The listing builds one solid part. Answer for the finished solid, in the listing's coordinates (mm). Face numbers are marked on the shaded views. A direction names the side the tool comes from. Coordinates: 2 decimals unless noted, no trailing zeros. Write each loop counter-clockwise with the first axis right and the second up, starting at its lowest first coordinate (ties: lowest second). Pieces come first, ordered by that corner, then holes. Notation, with made-up numbers: M 65,49.5 L 72,49.5 A6 ccw 72,58.5 Z; hole C 63.5,-7.5 d8. An arc over 180 degrees is marked long. Put each result on its own line as item: value. Start each with the question number.
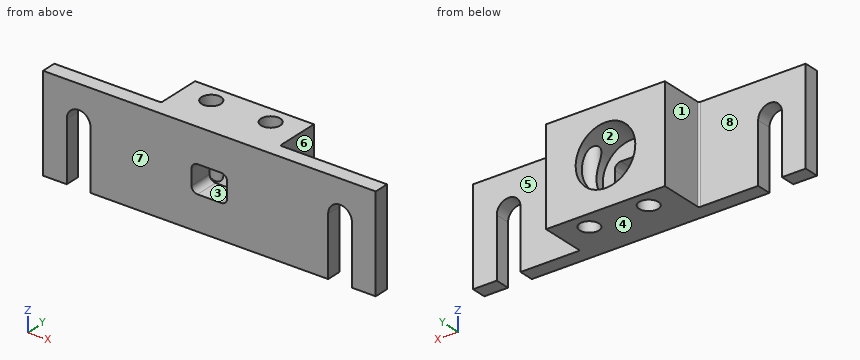
```python
from build123d import *

# Parameters (mm, degrees)
SKETCH1_W           = 28
SKETCH1_H           = 8
BOSS_EXTRUDE1_DEPTH = 1.25
SKETCH2_W           = 10
SKETCH2_H           = 8
BOSS_EXTRUDE2_DEPTH = 3.75
SKETCH3_R           = 2.51
CUT_EXTRUDE1_DEPTH  = 3
SKETCH4_W           = 3
SKETCH4_H           = 2.3
CUT_EXTRUDE2_DEPTH  = 15.866068747
CUT_EXTRUDE4_DEPTH  = 16.035374954
SKETCH7_R           = 0.81
CUT_EXTRUDE5_DEPTH  = 17.881943016
FILLET1_R           = 0.5
FILLET2_R           = 0.127


with BuildPart() as part:
    # Sketch1 → Boss-Extrude1 (new body)
    with BuildSketch(Plane(origin=(0, 0, 0), x_dir=(1, 0, 0), z_dir=(0, 1, 0))):
        Rectangle(SKETCH1_W, SKETCH1_H)
    extrude(amount=BOSS_EXTRUDE1_DEPTH)

    # Sketch2 → Boss-Extrude2 (add)
    with BuildSketch(Plane(origin=(0, 1.25, 0), x_dir=(1, 0, 0), z_dir=(0, 1, 0))):
        Rectangle(SKETCH2_W, SKETCH2_H)
    extrude(amount=BOSS_EXTRUDE2_DEPTH)

    # Sketch3 → Cut-Extrude1 (cut)
    with BuildSketch(Plane(origin=(0, 5, 0), x_dir=(1, 0, 0), z_dir=(0, 1, 0))):
        with Locations(Location((0, 0, 0), (0, 0, 270))):
            Circle(SKETCH3_R)
    extrude(amount=-CUT_EXTRUDE1_DEPTH, mode=Mode.SUBTRACT)

    # Sketch4 → Cut-Extrude2 (cut, through all)
    with BuildSketch(Plane(origin=(0, 2, 0), x_dir=(1, 0, 0), z_dir=(0, 1, 0))):
        Rectangle(SKETCH4_W, SKETCH4_H)
    extrude(amount=-CUT_EXTRUDE2_DEPTH, mode=Mode.SUBTRACT)

    # Sketch6 → Cut-Extrude4 (cut, through all)
    with BuildSketch(Plane(origin=(0, 1.25, 0), x_dir=(1, 0, 0), z_dir=(0, 1, 0))):
        with BuildLine():
            Line((12, 4), (12, -1))
            ThreePointArc((12, -1), (11, -2), (10, -1))
            Line((10, -1), (10, 4))
            Line((10, 4), (12, 4))
        make_face()
        with BuildLine():
            Line((-12, 4), (-12, -1))
            ThreePointArc((-12, -1), (-11, -2), (-10, -1))
            Line((-10, -1), (-10, 4))
            Line((-10, 4), (-12, 4))
        make_face()
    extrude(amount=-CUT_EXTRUDE4_DEPTH, mode=Mode.SUBTRACT)

    # Sketch7 → Cut-Extrude5 (cut, through all)
    with BuildSketch(Plane(origin=(0, 0, -4), x_dir=(-1, 0, 0), z_dir=(0, 0, -1))):
        with Locations((2.5, 3.5)):
            Circle(SKETCH7_R)
    cut_extrude5 = extrude(amount=-CUT_EXTRUDE5_DEPTH, mode=Mode.SUBTRACT)

    # Mirror1: Cut-Extrude5 across plane
    add(cut_extrude5.mirror(Plane.ZY), mode=Mode.SUBTRACT)

    # Fillet1
    fillet1_edges = [part.edges().sort_by_distance(p)[0] for p in [
        (-1.5, 1, -1.15),
        (1.5, 1, -1.15),
        (1.5, 1, 1.15),
        (-1.5, 1, 1.15),
    ]]
    fillet(fillet1_edges, radius=FILLET1_R)

    # Fillet2
    fillet2_edges = [part.edges().sort_by_distance(p)[0] for p in [
        (5, 1.25, 0),
        (-5, 1.25, 0),
    ]]
    fillet(fillet2_edges, radius=FILLET2_R)


solid = part.part
```
1) Determine the mould class of the marked faces 6, 7 and 8 for opening direction Y: +Y half, -Y half, draft (parallel to the pull), parting line (faces both ways), or undercut.
2) A cutting plane is placed at D-D on y = 3.5. Write down the section's boundary in (x, z).
3) Straight lines are drawn through the part: probe 1 along X at (y, z) = (0.35, -1.5); probe 2 along Y at (x, z) = (2.5, 0.5); probe 3 along X at (y, z) = (2.6, 0). For each, find the intervals that lie inside material, in ascending order.
4) For the marked faces 1, 2, 3, 4 and 5, determine the directions among +Z, -Z, +X, -X, +Y, -Y from which every point of the face is accessible in a straight line to the end or side of a thin tool.
5) Given pin 1 Ø3 at (y, z) = (3.5, -1) entering from +X; pin 2 Ø1.3 at (x, y) = (2.5, 3.5) entering from +Z; pin 3 Ø2.5 at (x, z) = (-9.5, 1.5) entering from +Y; pin 4 Ø1.5 at (x, z) = (-1, 0) entering from +Y, each flat-ended and moving along its own axis, determine where each tip first touches the part or whether it passes through.
6) A cutting plane is placed at A-A on z = -2.75. Write down the section's boundary in (x, y), then the cut area to 3 significant figures.
7) A cutting plane is placed at B-B on z = -1.5. Write down the section's boundary in (x, y).
8) A cutting plane is placed at C-C on x = 1.25. Write down the section's boundary in (y, z), then the cut area to 3 significant figures.
Answers follow:
1. face 6: draft
1. face 7: -Y half
1. face 8: +Y half
2. outline: M -5,-4 L -3.31,-4 L -3.31,4 L -5,4 Z; M -1.69,-4 L 1.69,-4 L 1.69,-1.86 A2.51 cw -1.69,-1.86 Z; M -1.69,1.86 A2.51 cw 1.69,1.86 L 1.69,4 L -1.69,4 Z; M 3.31,-4 L 5,-4 L 5,4 L 3.31,4 Z
3. probe 1: x = -14 to -12, -10 to 10, 12 to 14
3. probe 2: y = 0 to 2.69, 4.31 to 5
3. probe 3: x = -5 to -2.51, 2.51 to 5
4. face 1: +Z, -Z, -X, +Y
4. face 2: +Y
4. face 3: +Y, -Y
4. face 4: -Z, +X, -X, +Y, -Y
4. face 5: +Z, -Z, +X, +Y
5. pin 1: stops at x = 5
5. pin 2: passes through
5. pin 3: stops at y = 1.25
5. pin 4: stops at y = 2
6. outline: M -14,0 L -12,0 L -12,1.25 L -14,1.25 Z; M -10,0 L 10,0 L 10,1.25 L 5.13,1.25 A0.13 cw 5,1.38 L 5,5 L -5,5 L -5,1.38 A0.13 cw -5.13,1.25 L -10,1.25 Z; M 12,0 L 14,0 L 14,1.25 L 12,1.25 Z; hole C -2.5,3.5 d1.62; hole C 2.5,3.5 d1.62
6. area: 63.4 mm²
7. outline: M -14,0 L -12,0 L -12,1.25 L -14,1.25 Z; M -10,0 L 10,0 L 10,1.25 L 5.13,1.25 A0.13 cw 5,1.38 L 5,5 L 2.01,5 L 2.01,4.15 A0.81 cw long 2.01,2.85 L 2.01,2 L -2.01,2 L -2.01,2.85 A0.81 cw long -2.01,4.15 L -2.01,5 L -5,5 L -5,1.38 A0.13 cw -5.13,1.25 L -10,1.25 Z; M 12,0 L 14,0 L 14,1.25 L 12,1.25 Z
8. outline: M 0,-4 L 5,-4 L 5,-2.18 L 2,-2.18 L 2,-1.08 L 0,-1.08 Z; M 0,1.08 L 2,1.08 L 2,2.18 L 5,2.18 L 5,4 L 0,4 Z
8. area: 22.6 mm²
